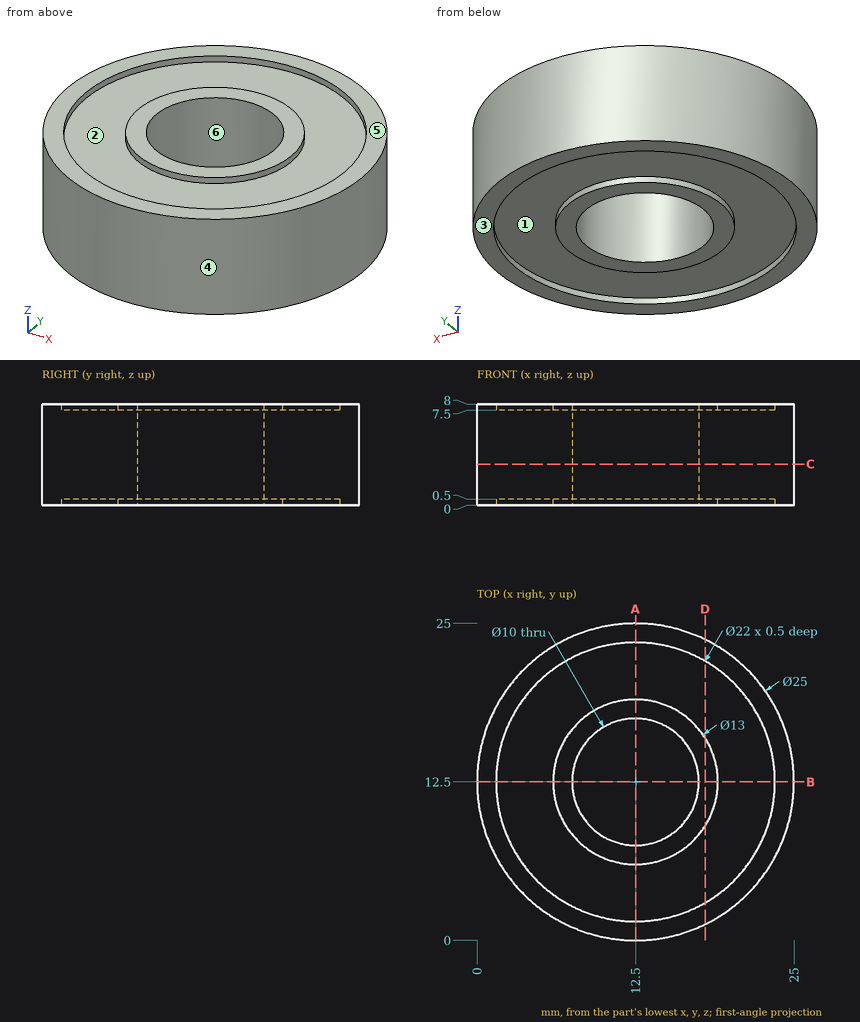
Check sheet for the drawn part. Datum: minimum x, y, z corner. Units: mm. A direction names the side the tool comes from. Give positions to 0.01 mm unless a question says otherwise; leave off trailing zeros. Order: outer loops, then holes, each group sorted by start corner. A loop starts at its lowest first (then second) coordinate and runs counter-clockwise, first axis right, second up. Notation, with made-up numbers: (-16.75, 52) -> (-11.75, 52) arc R24 ccw to (-11.75, 88) -> close; hole circle Ø3 at (-11, 41.25). An arc over 180 degrees is marked (long way). Return JSON: item names as keys, results as strings.
1. Mould release check, pull along Y, two halves, no side actions. Record for the marked faces 4, 5 and 6: +Y half, -Y half, draft (parallel to the pull), parting line (faces both ways), or undercut.
From the geometry:
{"face 4": "parting line", "face 5": "draft", "face 6": "undercut"}
2. Go/stop test with flat-tipped pins: P1, Ø3, axis at y = 20, z = 4.5, coming from the -X side; P2, Ø2, axis at x = 17.5, z = 1.5, coming from the +Y side; P3, Ø2, axis at x = 21.5, z = 6, coming from the +Y side. Record where each tip stops, or that it passes through.
From the geometry:
{"P1": "x = 1.53", "P2": "y = 24.34", "P3": "y = 22.1"}
3. Cross-section at C-C, the plane z = 3.25. Record the cut outline in (x, y).
From the geometry:
{"outline": "circle Ø25 at (12.5, 12.5); hole circle Ø10 at (12.5, 12.5)"}
4. Set-up check for the marked faces 1, 2 and 3: record each of +Z, -Z, +X, -X, +Y, -Y from which the full face is reachable in a straight line by a thin tool's end or side.
From the geometry:
{"face 1": "-Z", "face 2": "+Z", "face 3": "-Z, +X, -X, +Y, -Y"}
5. Cross-section at A-A, the plane x = 12.5. Record the cut outline in (y, z).
From the geometry:
{"outline": "(0, 0) -> (1.5, 0) -> (1.5, 0.5) -> (6, 0.5) -> (6, 0) -> (7.5, 0) -> (7.5, 8) -> (6, 8) -> (6, 7.5) -> (1.5, 7.5) -> (1.5, 8) -> (0, 8) -> close; (17.5, 0) -> (19, 0) -> (19, 0.5) -> (23.5, 0.5) -> (23.5, 0) -> (25, 0) -> (25, 8) -> (23.5, 8) -> (23.5, 7.5) -> (19, 7.5) -> (19, 8) -> (17.5, 8) -> close"}
6. Cross-section at D-D, the plane x = 18. Record the cut outline in (y, z), plus the area to 3 significant figures.
From the geometry:
{"outline": "(1.28, 0) -> (2.97, 0) -> (2.97, 0.5) -> (9.04, 0.5) -> (9.04, 0) -> (15.96, 0) -> (15.96, 0.5) -> (22.03, 0.5) -> (22.03, 0) -> (23.72, 0) -> (23.72, 8) -> (22.03, 8) -> (22.03, 7.5) -> (15.96, 7.5) -> (15.96, 8) -> (9.04, 8) -> (9.04, 7.5) -> (2.97, 7.5) -> (2.97, 8) -> (1.28, 8) -> close", "area": "167 mm^2"}
7. Material ranges on probe 1 along Y at (x, z) = (12.5, 1.5); probe 2 along Y at (x, z) = (12.5, 7.85); probe 3 along X at (y, z) = (10, 7.75), recorded low to high. Write a range as [from, to].
From the geometry:
{"probe 1": "[0, 7.5], [17.5, 25]", "probe 2": "[0, 1.5], [6, 7.5], [17.5, 19], [23.5, 25]", "probe 3": "[0.25, 1.79], [6.5, 8.17], [16.83, 18.5], [23.21, 24.75]"}
